Work out the finished part from the listing and answer in its coordinate system (mm). A direction names the side the tool comes from. Coordinates: 2 decimals unless noted, no trailing zeros. Order: outer loops, then holes, each group sorted by start corner. A loop starts at its lowest first (then second) coordinate and runs counter-clockwise, first axis right, second up. Notation, with made-up numbers: (48.25, 21) - (54.25, 21) arc R13 ccw to (54.25, 30) - close; hole circle Ø8 at (80, -24). An arc over 180 degrees is marked (long way). Answer as a JSON object with one key per item and string values. Group by question number.
1) Each of these flat-tipped pins is pushed along its axis until it touches: P1, Ø1, axis at y = -16, z = -11.5, coming from the -X side; P2, Ø4, axis at x = -17.5, z = -2.5, coming from the +Y side; P3, Ø4, axis at y = -9.5, z = -11, coming from the -X side; P4, Ø0.8, axis at x = -26, z = -11, coming from the +Y side. Where does it stop, or does it pass through?
2) Section D-D (x = -12) is taken. Give the vertices of the cut face in (y, z), plus the area to 3 significant figures.
3) A tool of negligible diameter and unlimited length cuts with its end or side. For faces 4 (the face through (-23.852, -20.913, -5.127)), 5 (the face through (33, -22, -4)), 6 (the face through (1, 1, -1.7)), 7 (the face through (-13.49, -15.11, 0.89)), 8 (the face through (-27, -22, -4)), from which of +Z, -Z, +X, -X, +Y, -Y can it reach the whole face along a straight path? Write none if from no direction.
4) Section A-A (z = -11) is taken. Give the vertices of the cut face in (x, y).
5) Find the intervals of material crossed by line 1 along Y through (x, z) = (0, -0.6); line 2 along Y through (x, z) = (0, 1.2); line 3 along Z through (x, y) = (-23, -19.25), in increasing order.
6) The mould has two halves that part along X. Classify faces 1 (the face through (24.586, -9.263, 0.887)), 2 (the face through (3, -22.7, -4)), 3 (the face through (-27.4, -16, -4)): released by +X, released by -X, zero draft, split by the parting line, or undercut.
7) Section B-B (x = 0) is taken. Count the separate pieces of the cut face and the enclosed holes in it, plus the area to 3 significant figures.
8) Section C-C (y = -18) is taken. Give the vertices of the cut face in (x, z).
from build123d import *

# Parameters (mm, degrees)
SKETCH_R     = 1.2
PAD_DEPTH    = 1.8
PAD001_DEPTH = 10.4
SKETCH002_W  = 3
SKETCH002_H  = 5
PAD002_DEPTH = 0.5
SKETCH003_W  = 3
SKETCH003_H  = 0.5
PAD003_DEPTH = 4.1
PAD004_DEPTH = 3
SKETCH006_W  = 1
SKETCH006_H  = 3
PAD005_DEPTH = 2
SKETCH007_R  = 3
PAD006_DEPTH = 1.7
SKETCH008_R  = 1.202636
POCKET_DEPTH = 15.901


with BuildPart() as part:
    # Sketch → Pad (new body)
    with BuildSketch(Plane.XY):
        with BuildLine():
            Line((-24.9, -24.5), (31.6, -24.5))
            Line((31.6, -24.5), (31.6, -22.7))
            ThreePointArc((32.3, -22), (31.805025, -22.205025), (31.6, -22.7))
            Line((32.3, -22), (34.1, -22))
            Line((34.1, -22), (34.1, -10.6))
            Line((15.335508, -7.962823), (34.1, -10.6))
            Line((3.956369, 3.820621), (15.335508, -7.962823))
            ThreePointArc((3.956369, 3.820621), (0.095988, 5.499162), (-3.820621, 3.956369))
            Line((-16.493585, -8.28177), (-3.820621, 3.956369))
            Line((-27.4, -10.6), (-16.493585, -8.28177))
            Line((-27.4, -22), (-27.4, -10.6))
            Line((-25.6, -22), (-27.4, -22))
            ThreePointArc((-24.9, -22.7), (-25.105025, -22.205025), (-25.6, -22))
            Line((-24.9, -24.5), (-24.9, -22.7))
        make_face()
        Circle(SKETCH_R, mode=Mode.SUBTRACT)
        with BuildLine():
            Line((-21.347203, -22.7), (19.83589, -22.7))
            Line((5.150202, -7.492526), (19.83589, -22.7))
            ThreePointArc((5.150202, -7.492526), (-0.091003, -5.213584), (-5.40855, -7.308222))
            Line((-21.347203, -22.7), (-5.40855, -7.308222))
        make_face(mode=Mode.SUBTRACT)
    extrude(amount=PAD_DEPTH)

    # Sketch001 → Pad001 (new body)
    with BuildSketch(Plane(origin=(0, 0, 0), x_dir=(1, 0, 0), z_dir=(0, 0, -1))):
        with BuildLine():
            Line((-27.4, 22), (-25.6, 22))
            ThreePointArc((-25.6, 22), (-25.105025, 22.205025), (-24.9, 22.7))
            Line((-24.9, 24.5), (-24.9, 22.7))
            Line((31.6, 24.5), (-24.9, 24.5))
            Line((31.6, 24.5), (31.6, 22.7))
            ThreePointArc((31.6, 22.7), (31.805025, 22.205025), (32.3, 22))
            Line((32.3, 22), (34.1, 22))
            Line((34.1, 22), (34.1, 10.6))
            Line((32.300003, 10.6), (34.1, 10.6))
            Line((32.300003, 20.2), (32.300003, 10.6))
            ThreePointArc((29.8, 22.7), (30.532234, 20.932232), (32.300003, 20.2))
            Line((-23.1, 22.7), (29.8, 22.7))
            ThreePointArc((-25.6, 20.2), (-23.832233, 20.932233), (-23.1, 22.7))
            Line((-25.6, 10.6), (-25.6, 20.2))
            Line((-27.4, 10.6), (-25.6, 10.6))
            Line((-27.4, 22), (-27.4, 10.6))
        make_face()
    extrude(amount=PAD001_DEPTH)

    # Sketch002 → Pad002 (new body)
    with BuildSketch(Plane(origin=(0, -22.7, 0), x_dir=(-1, 0, 0), z_dir=(0, 1, 0))):
        with Locations((-2.4, -7.9)):
            Rectangle(SKETCH002_W, SKETCH002_H)
    extrude(amount=PAD002_DEPTH)

    # Sketch003 → Pad003 (new body)
    with BuildSketch(Plane(origin=(0, 0, -10.4), x_dir=(1, 0, 0), z_dir=(0, 0, -1))):
        with Locations((2.4, 22.45)):
            Rectangle(SKETCH003_W, SKETCH003_H)
    extrude(amount=PAD003_DEPTH)

    # Sketch005 → Pad004 (new body)
    with BuildSketch(Plane(origin=(0.9, 0, 0), x_dir=(0, -1, 0), z_dir=(-1, 0, 0))):
        Polygon((22.2, -14.5), (23.24, -14.5), (22.7, -15.9), (22.2, -15.9), align=None)
    extrude(amount=-PAD004_DEPTH)

    # Sketch006 → Pad005 (new body)
    with BuildSketch(Plane(origin=(0, 0, -10.4), x_dir=(1, 0, 0), z_dir=(0, 0, -1))):
        with Locations((-26.1, 15.7)):
            Rectangle(SKETCH006_W, SKETCH006_H)
        with Locations((32.800003, 15.7)):
            Rectangle(SKETCH006_W, SKETCH006_H)
    extrude(amount=PAD005_DEPTH)

    # Sketch007 → Pad006 (new body)
    with BuildSketch(Plane(origin=(0, 0, 0), x_dir=(1, 0, 0), z_dir=(0, 0, -1))):
        Circle(SKETCH007_R)
    extrude(amount=PAD006_DEPTH)

    # Sketch008 → Pocket (cut, through all)
    with BuildSketch(Plane.XY):
        Circle(SKETCH008_R)
    extrude(amount=-POCKET_DEPTH, mode=Mode.SUBTRACT)


solid = part.part
Report:
{
 "1": {"P1": "stops at x = -26.6", "P2": "stops at y = -22.7", "P3": "stops at x = -27.4", "P4": "stops at y = -14.2"},
 "2": {"outline": "(-24.5, -10.4) - (-22.7, -10.4) - (-22.7, 1.8) - (-24.5, 1.8) - close; (-13.67, 0) - (-3.94, 0) - (-3.94, 1.8) - (-13.67, 1.8) - close", "area": "39.5 mm²"},
 "3": {"face 4": "-Z, +Y", "face 5": "+Z, -Z, +X, -Y", "face 6": "-Z, +X, -X, +Y", "face 7": "+Z, -Z", "face 8": "+Z, -Z, -X, -Y"},
 "4": {"outline": "(-26.6, -17.2) - (-25.6, -17.2) - (-25.6, -14.2) - (-26.6, -14.2) - close; (0.9, -22.7) - (3.9, -22.7) - (3.9, -22.2) - (0.9, -22.2) - close; (32.3, -17.2) - (33.3, -17.2) - (33.3, -14.2) - (32.3, -14.2) - close"},
 "5": {"line 1": "y = -24.5 to -22.7, -3 to -1.2, 1.2 to 3", "line 2": "y = -24.5 to -22.7, -5.22 to -1.2, 1.2 to 5.5", "line 3": "z = 0 to 1.8"},
 "6": {"face 1": "released by +X", "face 2": "undercut", "face 3": "released by -X"},
 "7": {"separate pieces": "3", "enclosed holes": "0", "area": "43.0 mm²"},
 "8": {"outline": "(-27.4, -10.4) - (-25.6, -10.4) - (-25.6, 0) - (-16.48, 0) - (-16.48, 1.8) - (-27.4, 1.8) - close; (15.3, 0) - (32.3, 0) - (32.3, -10.4) - (34.1, -10.4) - (34.1, 1.8) - (15.3, 1.8) - close"}
}
